For this review, take the finished solid that the model builds, in its own axes (mm). A direction names the side the tool comes from. Coordinates: 2 decimals unless noted, no trailing zeros. Loops run counter-clockwise (first coordinate to the right, second up) from the corner with the lowest first, then second, coordinate; pieces in that order, holes last. Notation, with made-up numbers: M 46.25,5.5 L 69.25,5.5 A10 cw 69.25,22.5 Z; hole C 29.25,52 d4. An arc over 180 degrees is marked long. Use one line per item in the form item = value.
```python
from build123d import *

# Parameters (mm, degrees)
BOSS_EXTRUDE1_DEPTH = 8.001
SKETCH2_R           = 6.35
BOSS_EXTRUDE2_DEPTH = 25.4


with BuildPart() as part:
    # Sketch1 → Boss-Extrude1 (new, symmetric)
    with BuildSketch(Plane.XY):
        with BuildLine():
            Line((-10.287, 0), (10.287, 0))
            Line((10.287, 0), (10.287, -18.161))
            ThreePointArc((10.287, -18.161), (0, -28.448), (-10.287, -18.161))
            Line((-10.287, -18.161), (-10.287, 0))
        make_face()
    extrude(amount=BOSS_EXTRUDE1_DEPTH, both=True)

    # Sketch2 → Boss-Extrude2 (add)
    with BuildSketch(Plane.XY.offset(8.001)):
        with Locations((0, -18.161)):
            Circle(SKETCH2_R)
    extrude(amount=BOSS_EXTRUDE2_DEPTH)


solid = part.part
```
1. For pin 1 Ø2 at (x, z) = (3, 13) entering from +Y; pin 2 Ø12 at (x, z) = (-4.5, 26.5) entering from +Y; pin 3 Ø3 at (y, z) = (-13.5, 13) entering from +X; pin 4 Ø8 at (y, z) = (-5.5, 28) entering from -X, all flat-tipped, find the tip position at first contact; note any pin that passes through.
Computed values:
pin_1 = -12.13
pin_2 = -11.81
pin_3 = 5.51
pin_4 = through
2. Consider section B-B on y = -23.75. Write out the cut boundary in (x, z).
Computed values:
outline = M -8.64,-8 L 8.64,-8 L 8.64,8 L 3.01,8 L 3.01,33.4 L -3.01,33.4 L -3.01,8 L -8.64,8 Z
3. Consider section D-D on y = -8. Write out the cut boundary in (x, z).
Computed values:
outline = M -10.29,-8 L 10.29,-8 L 10.29,8 L -10.29,8 Z
4. Tool access review of faces 1 (the face through (0, -11, 8.001)), 2 (the face through (0, -14, -8.001)): name each direction out of +Z, -Z, +X, -X, +Y, -Y from which nothing blocks a thin tool from reaching the whole face with its end or side.
Computed values:
face_1 = +Z
face_2 = -Z, +X, -X, +Y, -Y
5. Wall thickness on line 1 along Z through (x, y) = (-6.25, -5.5); line 2 along X through (y, z) = (-18.5, 8.5); line 3 along X through (y, z) = (-23.5, 10.5): over which ranges is each line inside the solid? List them lowest first. Write a range as from..to.
Computed values:
line_1 = -8..8
line_2 = -6.34..6.34
line_3 = -3.44..3.44
6. Consider section A-A on x = 0. Write out the cut boundary in (y, z).
Computed values:
outline = M -28.45,-8 L 0,-8 L 0,8 L -11.81,8 L -11.81,33.4 L -24.51,33.4 L -24.51,8 L -28.45,8 Z
7. Consider section C-C on z = 30.5. Write out the cut boundary in (x, y), plus the area to 3 significant figures.
Computed values:
outline = C 0,-18.16 d12.7
area = 127 mm2
